from build123d import *

# Parameters (mm, degrees)
BOSS_EXTRUDE1_DEPTH      = 10
BOSS_EXTRUDE1_DEPTH_BACK = 10
SKETCH1_R                = 19.05
FILLET1_R                = 1
SKETCH2_R                = 12.5
CUT_EXTRUDE1_DEPTH       = 2
CUT_EXTRUDE2_START       = -2
SKETCH3_R                = 12.5
CUT_EXTRUDE2_DEPTH       = 2
SKETCH4_R                = 6
SKETCH4_R_2              = 4
BOSS_EXTRUDE2_DEPTH      = 1
SKETCH5_R                = 3.5
BOSS_EXTRUDE3_DEPTH      = 8
CHAMFER1_SIZE            = 0.5


with BuildPart() as part:
    # Sketch1 → Boss-Extrude1 (new, two sides: drawn at the far end of the back side and taken through both)
    with BuildSketch(Plane.XY.offset(-BOSS_EXTRUDE1_DEPTH_BACK)):
        Circle(SKETCH1_R)
    extrude(amount=BOSS_EXTRUDE1_DEPTH + BOSS_EXTRUDE1_DEPTH_BACK)

    # Fillet1
    fillet1_edges = [part.edges().sort_by_distance(p)[0] for p in [
        (-19.05, 0, -10),
        (-19.05, 0, 10),
    ]]
    fillet(fillet1_edges, radius=FILLET1_R)

    # Sketch2 → Cut-Extrude1 (cut)
    with BuildSketch(Plane.XY.offset(10)):
        Circle(SKETCH2_R)
    extrude(amount=-CUT_EXTRUDE1_DEPTH, mode=Mode.SUBTRACT)

    # Sketch3 → Cut-Extrude2 (cut)
    with BuildSketch(Plane(origin=(0, 0, -10), x_dir=(-1, 0, 0), z_dir=(0, 0, -1)).offset(CUT_EXTRUDE2_START)):
        with Locations(Location((0, 0, 0), (0, 0, 180))):
            Circle(SKETCH3_R)
    extrude(amount=CUT_EXTRUDE2_DEPTH, mode=Mode.SUBTRACT)

    # Sketch4 → Boss-Extrude2 (add)
    with BuildSketch(Plane.XY.offset(8)):
        Circle(SKETCH4_R)
        Circle(SKETCH4_R_2, mode=Mode.SUBTRACT)
    boss_extrude2 = extrude(amount=BOSS_EXTRUDE2_DEPTH)

    # Mirror1: Boss-Extrude2 across plane
    add(boss_extrude2.mirror(Plane.XY))

    # Sketch5 → Boss-Extrude3 (add)
    with BuildSketch(Plane.XY.offset(8)):
        Circle(SKETCH5_R)
    boss_extrude3 = extrude(amount=BOSS_EXTRUDE3_DEPTH)

    # Mirror2: Boss-Extrude3 across plane
    add(boss_extrude3.mirror(Plane.XY))

    # Chamfer1
    chamfer1_edges = [part.edges().sort_by_distance(p)[0] for p in [
        (-3.5, 0, 16),
        (-3.5, 0, -16),
    ]]
    chamfer(chamfer1_edges, length=CHAMFER1_SIZE)


solid = part.part
Design review of the part built by this model. Coordinates are the model's own, in mm. A direction names the side the tool comes from. Round coordinates to 2 decimals unless told otherwise and drop trailing zeros. Order: outer loops, then holes, each group sorted by start corner. A loop starts at its lowest first (then second) coordinate and runs counter-clockwise, first axis right, second up.
1) Draft analysis for pull direction Y (two halves, no side actions). For faces 1 (the cylindrical face through (-15.12, -11.59, -0.13)), 2 (the flat face through (0, 0, -16)), 3 (the cylindrical face through (3.233, -1.341, 11.698)), state which applies: released by +Y, released by -Y, zero draft, split by the parting line, or undercut.
The answers:
face 1: split by the parting line
face 2: zero draft
face 3: undercut
2) For L1, parallel to Y at x = 0, z = 8.5; L2, parallel to Y at x = 0, z = -9.2; L3, parallel to Z at x = 11, y = -11, list the stretches that pass through material, from the lowest coordinate up.
The answers:
L1: y = -19.05 to -12.5, -6 to -4, -3.5 to 3.5, 4 to 6, 12.5 to 19.05
L2: y = -19.03 to -12.5, -3.5 to 3.5, 12.5 to 19.03
L3: z = -10 to 10
3) Machinability: for faces 4 (the flat face through (0, 0, 16)), 5 (the cylindrical face through (-5.994, 0.264, 8.493)), 6 (the cylindrical face through (11.923, -3.755, -8.986)), which of the approach directions +Z, -Z, +X, -X, +Y, -Y give a long, thin tool a straight path to every point of the face, cutting with its end or side? Answer none if there is none.
The answers:
face 4: +Z, +X, -X, +Y, -Y
face 5: +Z
face 6: -Z
4) Clearance check with flat-ended pins moving along their axes: pin 1 Ø10 at (x, z) = (-10, -3.5) entering from +Y; pin 2 Ø8 at (x, y) = (-4, -15) entering from +Z; pin 3 Ø10 at (x, z) = (5.5, 13) entering from -Y. State where each tip first meets the part, or that it passes through.
The answers:
pin 1: stops at y = 18.38
pin 2: stops at z = 10
pin 3: stops at y = -18.9
5) Consider section A-A (z = 2.5). State the section outline as (x, y) points, plus the area to 3 significant figures.
The answers:
outline: circle Ø38.1 at (0, 0)
area: 1,140 mm2
